The listing builds one solid part. Answer for the finished solid, in the listing's coordinates (mm). Face numbers are marked on the shaded views. Give positions to 0.01 mm unless a question says otherwise; leave off trailing zeros. Loops run counter-clockwise (first coordinate to the right, second up) from the corner with the lowest first, then second, coordinate; pieces in that order, holes last.
Item 1: Consider line 1 along X through (y, z) = (0.9, -27); line 2 along X through (y, z) = (0.5, -4); line 3 along Z through (x, y) = (3.75, 1.05). Determine where each line is inside the solid, lowest interval first.
Item 2: The mould has two halves that part along X. Classify the marked faces 1 and 2: pulls with the +X half, pulls with the -X half, needs draft (parallel to the pull), parting line crosses it, or undercut.
Item 3: Each of these flat-tipped pins is pushed along its axis until it touches: pin 1 Ø6 at (x, z) = (8.5, -21) entering from +Y; pin 2 Ø2 at (x, z) = (2.5, -3.5) entering from +Y; pin 3 Ø2.5 at (x, z) = (12, -29) entering from +Y. Where does it stop, or does it pass through?
Item 4: Section A-A, the plane y = 1.65 is taken. Give the vertices of the cut face in (x, z).
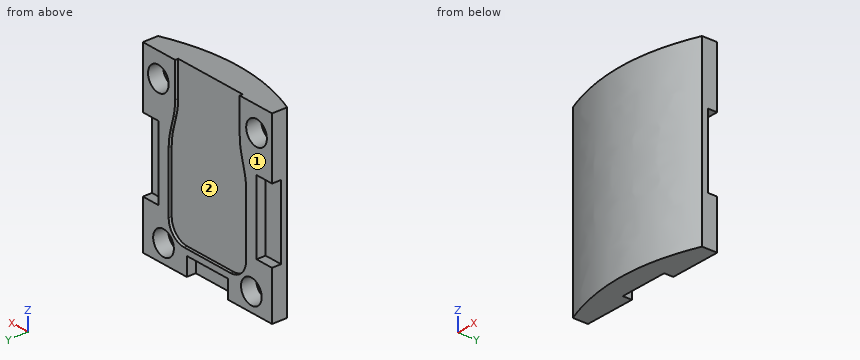
from build123d import *

# Parameters (mm, degrees)
SKETCH1_W           = 25
SKETCH1_H           = 30
BOSS_EXTRUDE1_DEPTH = 2.5
CUT_EXTRUDE1_DEPTH  = 0.5
SKETCH3_R           = 2
CUT_EXTRUDE2_DEPTH  = 3.5
BOSS_EXTRUDE2_DEPTH = 30
SKETCH5_W           = 8
SKETCH5_H           = 3
SKETCH5_W_2         = 3
SKETCH5_H_2         = 12
CUT_EXTRUDE3_DEPTH  = 1.5


with BuildPart() as part:
    # Sketch1 → Boss-Extrude1 (new body)
    with BuildSketch(Plane(origin=(0, 0, 0), x_dir=(1, 0, 0), z_dir=(0, 1, 0))):
        with Locations((12.5, 15)):
            Rectangle(SKETCH1_W, SKETCH1_H)
    extrude(amount=BOSS_EXTRUDE1_DEPTH)

    # Sketch2 → Cut-Extrude1 (cut)
    with BuildSketch(Plane(origin=(0, 2.5, 0), x_dir=(1, 0, 0), z_dir=(0, 1, 0))):
        with BuildLine():
            Line((8, 26), (17, 26))
            ThreePointArc((17, 26), (19.121320344, 25.121320344), (20, 23))
            Line((20, 23), (20, 13))
            ThreePointArc((20, 13), (19.915325472, 11.701415851), (19.662735842, 10.424823102))
            Line((19.662735842, 10.424823102), (19.087264158, 8.265503148))
            ThreePointArc((19.087264158, 8.265503148), (18.834674528, 6.988910399), (18.75, 5.690326251))
            Line((18.75, 5.690326251), (18.75, 0))
            Line((18.75, 0), (6.25, 0))
            Line((6.25, 0), (6.25, 5.690326251))
            ThreePointArc((6.25, 5.690326251), (6.165325472, 6.988910399), (5.912735842, 8.265503148))
            Line((5.912735842, 8.265503148), (5.337264158, 10.424823102))
            ThreePointArc((5.337264158, 10.424823102), (5.084674528, 11.701415851), (5, 13))
            Line((5, 13), (5, 23))
            ThreePointArc((5, 23), (5.878679656, 25.121320344), (8, 26))
        make_face()
    extrude(amount=-CUT_EXTRUDE1_DEPTH, mode=Mode.SUBTRACT)

    # Sketch3 → Cut-Extrude2 (cut)
    with BuildSketch(Plane(origin=(0, 2.5, 0), x_dir=(1, 0, 0), z_dir=(0, 1, 0))):
        with Locations((21, 27)):
            Circle(SKETCH3_R)
        with Locations((4, 27)):
            Circle(SKETCH3_R)
        with Locations((3, 4)):
            Circle(SKETCH3_R)
        with Locations((22, 4)):
            Circle(SKETCH3_R)
    extrude(amount=-CUT_EXTRUDE2_DEPTH, mode=Mode.SUBTRACT)

    # Sketch4 → Boss-Extrude2 (add)
    with BuildSketch(Plane.XY):
        with BuildLine():
            Line((25, 0), (0, 0))
            add(Edge.make_bspline(
                [(25, 0), (12.5, -5), (0, 0)],
                knots=[0, 0, 0, 1, 1, 1], degree=2))
        make_face()
    extrude(amount=-BOSS_EXTRUDE2_DEPTH)

    # Sketch5 → Cut-Extrude3 (cut)
    with BuildSketch(Plane(origin=(0, 2.5, 0), x_dir=(1, 0, 0), z_dir=(0, 1, 0))):
        with Locations((12.5, 28.5)):
            Rectangle(SKETCH5_W, SKETCH5_H)
        with Locations((23.5, 16)):
            Rectangle(SKETCH5_W_2, SKETCH5_H_2)
        with Locations((1.5, 16)):
            Rectangle(SKETCH5_W_2, SKETCH5_H_2)
    extrude(amount=-CUT_EXTRUDE3_DEPTH, mode=Mode.SUBTRACT)


solid = part.part
Worked answers:
1. line 1: x = 0 to 2, 6 to 19, 23 to 25
1. line 2: x = 0 to 1, 5 to 20, 24 to 25
1. line 3: z = -30 to -28.98, -25.02 to -5.85, -2.15 to 0
2. face 1: needs draft
2. face 2: undercut
3. pin 1: stops at y = 2
3. pin 2: stops at y = 0
3. pin 3: stops at y = 1
4. outline: (0, -30) - (8.5, -30) - (8.5, -27) - (16.5, -27) - (16.5, -30) - (25, -30) - (25, -22) - (22, -22) - (22, -10) - (25, -10) - (25, 0) - (0, 0) - (0, -10) - (3, -10) - (3, -22) - (0, -22) - close; hole circle Ø4 at (3, -4); hole circle Ø4 at (4, -27); hole circle Ø4 at (21, -27); hole circle Ø4 at (22, -4)
